```python
from build123d import *

# Parameters (mm, degrees)
EXTRUDE_1_DEPTH     = 5
FILLET_4_R          = 5
FILLET_5_R          = 5
FILLET_6_R          = 5
FILLET_7_R          = 5
FILLET_8_R          = 3
FILLET_9_R          = 3
FILLET_10_R         = 3
FILLET_11_R         = 3
FILLET_12_R         = 5
FILLET_13_R         = 5
FILLET_14_R         = 5
FILLET_15_R         = 5
CUT_EXTRUDE_START   = -5
CUT_EXTRUDE_2_DEPTH = 5


# Read off the part's stored shape, not the designer's step: 切除-拉伸2
with BuildPart() as part:
    # 草图1 → 凸台-拉伸1 (new body)
    with BuildSketch(Plane.XY):
        Polygon((-75, 5), (-40, 5), (-40, 40), (-30, 40), (-30, 5), (30, 5), (30, 40), (40, 40), (40, 5), (75, 5), (75, -5), (-75, -5), align=None)
    extrude(amount=EXTRUDE_1_DEPTH)

    # 圆角4
    fillet_4_edges = [part.edges().sort_by_distance(p)[0] for p in [
        (-40, 40, 2.5),
    ]]
    fillet(fillet_4_edges, radius=FILLET_4_R)

    # 圆角5
    fillet_5_edges = [part.edges().sort_by_distance(p)[0] for p in [
        (-30, 40, 2.5),
    ]]
    fillet(fillet_5_edges, radius=FILLET_5_R - 0.0001)  # a hair under: the kernel refuses the full size

    # 圆角6
    fillet_6_edges = [part.edges().sort_by_distance(p)[0] for p in [
        (30, 40, 2.5),
    ]]
    fillet(fillet_6_edges, radius=FILLET_6_R)

    # 圆角7
    fillet_7_edges = [part.edges().sort_by_distance(p)[0] for p in [
        (40, 40, 2.5),
    ]]
    fillet(fillet_7_edges, radius=FILLET_7_R - 0.0001)  # a hair under: the kernel refuses the full size

    # 圆角8
    fillet_8_edges = [part.edges().sort_by_distance(p)[0] for p in [
        (-75, 5, 2.5),
    ]]
    fillet(fillet_8_edges, radius=FILLET_8_R)

    # 圆角9
    fillet_9_edges = [part.edges().sort_by_distance(p)[0] for p in [
        (-75, -5, 2.5),
    ]]
    fillet(fillet_9_edges, radius=FILLET_9_R)

    # 圆角10
    fillet_10_edges = [part.edges().sort_by_distance(p)[0] for p in [
        (75, 5, 2.5),
    ]]
    fillet(fillet_10_edges, radius=FILLET_10_R)

    # 圆角11
    fillet_11_edges = [part.edges().sort_by_distance(p)[0] for p in [
        (75, -5, 2.5),
    ]]
    fillet(fillet_11_edges, radius=FILLET_11_R)

    # 圆角12
    fillet_12_edges = [part.edges().sort_by_distance(p)[0] for p in [
        (40, 5, 2.5),
    ]]
    fillet(fillet_12_edges, radius=FILLET_12_R)

    # 圆角13
    fillet_13_edges = [part.edges().sort_by_distance(p)[0] for p in [
        (30, 5, 2.5),
    ]]
    fillet(fillet_13_edges, radius=FILLET_13_R)

    # 圆角14
    fillet_14_edges = [part.edges().sort_by_distance(p)[0] for p in [
        (-30, 5, 2.5),
    ]]
    fillet(fillet_14_edges, radius=FILLET_14_R)

    # 圆角15
    fillet_15_edges = [part.edges().sort_by_distance(p)[0] for p in [
        (-40, 5, 2.5),
    ]]
    fillet(fillet_15_edges, radius=FILLET_15_R)

    # 切除-拉伸2 outline → 切除-拉伸2 (cut)
    with BuildSketch(Plane.XY.offset(5).offset(CUT_EXTRUDE_START)):
        with BuildLine():
            ThreePointArc((-36.7, 6.7), (-36.202081528, 5.497918472), (-35, 5))
            Line((-35, 5), (-34.95, 5))
            ThreePointArc((-34.95, 5), (-33.783273811, 5.483273811), (-33.3, 6.65))
            Line((-33.3, 6.65), (-33.3, 34.25))
            ThreePointArc((-33.3, 34.25), (-33.797918472, 35.452081528), (-35, 35.95))
            Line((-35, 35.95), (-35.05, 35.95))
            ThreePointArc((-35.05, 35.95), (-36.216726189, 35.466726189), (-36.7, 34.3))
            Line((-36.7, 34.3), (-36.7, 6.7))
        make_face()
        with BuildLine():
            Line((-30.527301477, -0.05), (-30.527301477, 0.05))
            ThreePointArc((-30.527301477, 0.05), (-31.010575288, 1.216726189), (-32.177301477, 1.7))
            Line((-32.177301477, 1.7), (-68.351867054, 1.699998944))
            ThreePointArc((-68.351867054, 1.699998944), (-69.517386106, 1.216065899), (-70, 0.05))
            Line((-70, 0.05), (-70, -0.05))
            ThreePointArc((-70, -0.05), (-69.516726189, -1.216726189), (-68.35, -1.7))
            Line((-68.35, -1.7), (-32.177301477, -1.7))
            ThreePointArc((-32.177301477, -1.7), (-31.010575288, -1.216726189), (-30.527301477, -0.05))
        make_face()
        with BuildLine():
            Line((-24.310810244, -1.7), (21.867276161, -1.7))
            ThreePointArc((21.867276161, -1.7), (23.03400235, -1.216726189), (23.517276161, -0.05))
            Line((23.517276161, -0.05), (23.517276161, 0.05))
            ThreePointArc((23.517276161, 0.05), (23.03400235, 1.216726189), (21.867276161, 1.7))
            Line((21.867276161, 1.7), (-24.310810244, 1.7))
            ThreePointArc((-24.310810244, 1.7), (-25.477536433, 1.216726189), (-25.960810244, 0.05))
            Line((-25.960810244, 0.05), (-25.960810244, -0.05))
            ThreePointArc((-25.960810244, -0.05), (-25.477536433, -1.216726189), (-24.310810244, -1.7))
        make_face()
        with BuildLine():
            Line((29.696775282, -1.7), (68.35, -1.7))
            ThreePointArc((68.35, -1.7), (69.516726189, -1.216726189), (70, -0.05))
            Line((70, -0.05), (70, 0.05))
            ThreePointArc((70, 0.05), (69.516726189, 1.216726189), (68.35, 1.7))
            Line((68.35, 1.7), (29.696775282, 1.7))
            ThreePointArc((29.696775282, 1.7), (28.530049093, 1.216726189), (28.046775282, 0.05))
            Line((28.046775282, 0.05), (28.046775282, -0.05))
            ThreePointArc((28.046775282, -0.05), (28.530049093, -1.216726189), (29.696775282, -1.7))
        make_face()
        with BuildLine():
            ThreePointArc((36.800022997, 34.2), (36.302104525, 35.402081528), (35.100022997, 35.9))
            Line((35.100022997, 35.9), (35.050022997, 35.9))
            ThreePointArc((35.050022997, 35.9), (33.812569868, 35.387430132), (33.3, 34.149977003))
            Line((33.3, 34.149977003), (33.3, 6.65))
            ThreePointArc((33.3, 6.65), (33.797918472, 5.447918472), (35, 4.95))
            Line((35, 4.95), (35.150022997, 4.95))
            ThreePointArc((35.150022997, 4.95), (36.316749186, 5.433273812), (36.800022997, 6.6))
            Line((36.800022997, 6.6), (36.800022997, 34.2))
        make_face()
    extrude(amount=CUT_EXTRUDE_2_DEPTH, mode=Mode.SUBTRACT)


solid = part.part
```
Geometry: final body of the model. Coordinates: model frame, mm. A direction names the side the tool comes from. Round coordinates to 2 decimals unless told otherwise and drop trailing zeros. Write each loop counter-clockwise with the first axis right and the second up, starting at its lowest first coordinate (ties: lowest second). Pieces come first, ordered by that corner, then holes. Notation, with made-up numbers: M 34,6 L 76,6 A30 cw 76,32 Z; hole C 63,88 d11. An arc over 180 degrees is marked long. Answer in a Markdown table with one row per item. Add a question column.
(1) Contact query for flat-ended pins moving along their axis: pin 1 (2.5 mm diameter, centred on y = 19.5, z = 1.5, fed in from +X); pin 2 (6 mm diameter, centred on x = 27, y = 1, fed in from -Z); pin 3 (1.5 mm diameter, centred on x = -5, z = 3.5, fed in from +Y). Output: stop coordinate, or through.
(2) Draft query along X for faces 5 (the face through (-5, 3, 5)), 6 (the face through (-1, 1.7, 2)), 7 (the face through (-40, 22, 2)). Return one class per face: pulls with the +X half, pulls with the -X half, needs draft (parallel to the pull), parting line crosses it, or undercut.
(3) Cut plane D-D, the plane z = 2.95. Give the number of separate pieces and of enclosed holes in the cut face, then the cut area to 3 significant figures.
(4) Reachability of faces 1 (the face through (58, 5, 2)), 2 (the face through (29, 7, 3)), 3 (the face through (-50, 1.7, 2)), 4 (the face through (1, -5, 2)) from +Z, -Z, +X, -X, +Y, -Y: full face, straight path, thin tool, end or side. Return the list, or none.
(5) Cut plane A-A, the plane y = 32. Return the cut outline in (x, z), then the cut area to 3 significant figures.
(6) Ray query, L1, parallel to X at y = 11.5, z = 3.5; L2, parallel to X at y = 0, z = 3.35; L3, parallel to Y at x = -33.5, z = 2.8. Return the intervals inside material, ascending.
(7) Cut plane C-C, the plane x = 41.5. Return the cut outline in (y, z).
(8) Cut plane B-B, the plane x = -17.5. Return the cut outline in (y, z), then the cut area to 3 significant figures.
Established:
| question | item | result |
|---|---|---|
| 1 | pin 1 | x = 40 |
| 1 | pin 2 | z = 0 |
| 1 | pin 3 | y = 5 |
| 2 | face 5 | needs draft |
| 2 | face 6 | undercut |
| 2 | face 7 | pulls with the -X half |
| 3 | separate pieces | 1 |
| 3 | enclosed holes | 5 |
| 3 | area | 1,550 mm² |
| 4 | face 1 | +Z, -Z, +X, +Y |
| 4 | face 2 | +Z, -Z, +Y |
| 4 | face 3 | +Z, -Z |
| 4 | face 4 | +Z, -Z, +X, -X, -Y |
| 5 | outline | M -40,0 L -36.7,0 L -36.7,5 L -40,5 Z; M -33.3,0 L -30,0 L -30,5 L -33.3,5 Z; M 30,0 L 33.3,0 L 33.3,5 L 30,5 Z; M 36.8,0 L 40,0 L 40,5 L 36.8,5 Z |
| 5 | area | 65.5 mm² |
| 6 | L1 | -40 to -36.7, -33.3 to -30, 30 to 33.3, 36.8 to 40 |
| 6 | L2 | -75 to -70, -30.53 to -25.96, 23.52 to 28.05, 70 to 75 |
| 6 | L3 | -5 to -1.7, 1.7 to 5.86, 35.05 to 39.77 |
| 7 | outline | M -5,0 L -1.7,0 L -1.7,5 L -5,5 Z; M 1.7,0 L 6.43,0 L 6.43,5 L 1.7,5 Z |
| 8 | outline | M -5,0 L -1.7,0 L -1.7,5 L -5,5 Z; M 1.7,0 L 5,0 L 5,5 L 1.7,5 Z |
| 8 | area | 33.0 mm² |
